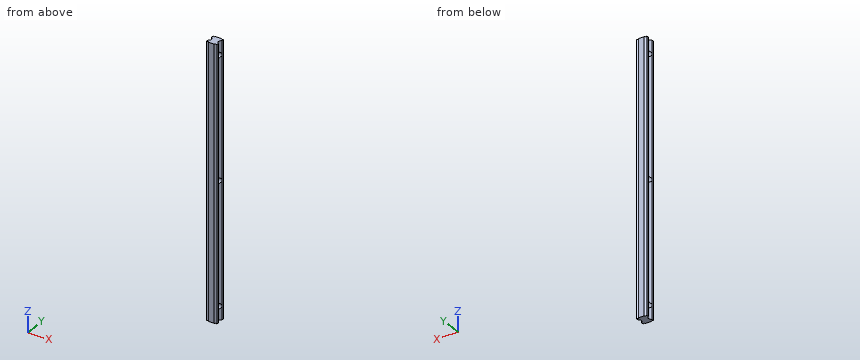
Autodesk Inventor part; units mm, degrees
ref_plane "to_ball_1_XY" through (1.2, -0.75, 109.375) normal (0, 0, 1) x (1, 0, 0)
ref_plane "to_ball_1_YZ" through (1.2, -0.75, 109.375) normal (1, 0, 0) x (0, 1, 0)
ref_plane "to_ball_1_ZX" through (1.2, -0.75, 109.375) normal (0, 1, 0) x (0, 0, 1)
sketch "Sketch_1" plane through (0, 0, 0) normal (0, 0, 1) x (1, 0, 0)
  line L0 (0, 2.9516) -> (0, 0.3457)
  arc A0 (2.6416, 0) -> (0, 0.3457) centre (1.2, -0.75) ccw
  line L1 (2.6416, 0) -> (8.7584, 0)
  arc A1 (11.4, 0.3457) -> (8.7584, 0) centre (10.2, -0.75) ccw
  line L2 (11.4, 0.3457) -> (11.4, 2.9516)
  arc A2 (11.4, 9.1484) -> (11.4, 2.9516) centre (12.8, 6.05) ccw
  line L3 (11.4, 9.1484) -> (11.4, 11.7543)
  arc A3 (8.7584, 12.1) -> (11.4, 11.7543) centre (10.2, 12.85) ccw
  line L4 (8.7584, 12.1) -> (2.6416, 12.1)
  arc A4 (0, 11.7543) -> (2.6416, 12.1) centre (1.2, 12.85) ccw
  line L5 (0, 11.7543) -> (0, 9.1484)
  arc A5 (0, 2.9516) -> (0, 9.1484) centre (-1.4, 6.05) ccw
extrude "Extrusion1" add sketch "Sketch_1" along normal blind 300
sketch "Sketch_3" plane through (0, 0, 15) normal (0, 0, 1) x (1, 0, 0)
  line L0 (11.4, 6.05) -> (0, 6.05)
  line L1 (0, 6.05) -> (0, 9.3)
  line L2 (0, 9.3) -> (11.4, 9.3)
  line L3 (11.4, 9.3) -> (11.4, 6.05)
  line L4 (11.4, 6.05) -> (0, 6.05)
revolve "Revolution1" cut sketch "Sketch_3" angle 360 about axis through (11.4, 6.05, 15) along (1, 0, 0)
pattern_linear "Rectangular Pattern1" count 3 spacing 135 along (0, 0, 1) of "Revolution1"
ref_plane "to_ball_1_XY" through (1.2, -0.75, 109.375) normal (0, 0, 1) x (1, 0, 0)
ref_plane "to_ball_1_YZ" through (1.2, -0.75, 109.375) normal (1, 0, 0) x (0, 1, 0)
ref_plane "to_ball_1_ZX" through (1.2, -0.75, 109.375) normal (0, 1, 0) x (0, 0, 1)
ref_plane "to_ball_2_XY" through (10.2, -0.75, 109.375) normal (0, 0, 1) x (1, 0, 0)
ref_plane "to_ball_2_YZ" through (10.2, -0.75, 109.375) normal (1, 0, 0) x (0, 1, 0)
ref_plane "to_ball_2_ZX" through (10.2, -0.75, 109.375) normal (0, 1, 0) x (0, 0, 1)
ref_plane "to_ball_3_XY" through (1.2, 12.85, 109.375) normal (0, 0, 1) x (1, 0, 0)
ref_plane "to_ball_3_YZ" through (1.2, 12.85, 109.375) normal (1, 0, 0) x (0, 1, 0)
ref_plane "to_ball_3_ZX" through (1.2, 12.85, 109.375) normal (0, 1, 0) x (0, 0, 1)
ref_plane "to_ball_4_XY" through (10.2, 12.85, 109.375) normal (0, 0, 1) x (1, 0, 0)
ref_plane "to_ball_4_YZ" through (10.2, 12.85, 109.375) normal (1, 0, 0) x (0, 1, 0)
ref_plane "to_ball_4_ZX" through (10.2, 12.85, 109.375) normal (0, 1, 0) x (0, 0, 1)
ref_plane "to_body_XY" through (5.6, 6.05, 150) normal (0, 0, 1) x (1, 0, 0)
ref_plane "to_body_YZ" through (5.6, 6.05, 150) normal (1, 0, 0) x (0, 1, 0)
ref_plane "to_body_ZX" through (5.6, 6.05, 150) normal (0, 1, 0) x (0, 0, 1)
ref_plane "to_body2_XY" through (5.8, 6.05, 150) normal (0, 0, 1) x (1, 0, 0)
ref_plane "to_body2_YZ" through (5.8, 6.05, 150) normal (1, 0, 0) x (0, 1, 0)
ref_plane "to_body2_ZX" through (5.8, 6.05, 150) normal (0, 1, 0) x (0, 0, 1)
properties part number "SAR330-30_r" material "Aluminum 6061"
Source: CAD feature listing. Evaluate the final solid. Frame: model axes, mm. Give positions to 0.01 mm unless a question says otherwise; leave off trailing zeros. Order: outer loops, then holes, each group sorted by start corner. A loop starts at its lowest first (then second) coordinate and runs counter-clockwise, first axis right, second up. Notation, with made-up numbers: (17.5, -11.75) -> (75.5, -11.75) arc R21 cw to (75.5, 11.25) -> close; hole circle Ø2 at (-5.5, -1). An arc over 180 degrees is marked (long way). Use a Markdown table: item, result.
Q1. First-contact query: P1, Ø5, axis at y = 6.05, z = 285, coming from the +X side. Flat tip, straight axial feed; report the tip coordinate or a pass-through.
A:
| item | result |
|---|---|
| P1 | through |
Q2. Section B-B (x = 6.5). Return the cut outline in (y, z).
A:
| item | result |
|---|---|
| outline | (0, 0) -> (12.1, 0) -> (12.1, 300) -> (0, 300) -> close; hole circle Ø6.5 at (6.05, 15); hole circle Ø6.5 at (6.05, 150); hole circle Ø6.5 at (6.05, 285) |
Q3. Material intervals for line 1 (Z direction, x = 7.25, y = 6.5); line 2 (Z direction, x = 9.25, y = 7.75); line 3 (Y direction, x = 6, z = 15), sorted ascending. Write a range as [from, to].
A:
| item | result |
|---|---|
| line 1 | [0, 11.78], [18.22, 146.78], [153.22, 281.78], [288.22, 300] |
| line 2 | [0, 12.23], [17.77, 147.23], [152.77, 282.23], [287.77, 300] |
| line 3 | [0, 2.8], [9.3, 12.1] |
Q4. Section A-A (y = 6.05). Return the cut outline in (x, z).
A:
| item | result |
|---|---|
| outline | (2, 0) -> (9.4, 0) -> (9.4, 11.75) -> (2, 11.75) -> close; (2, 18.25) -> (9.4, 18.25) -> (9.4, 146.75) -> (2, 146.75) -> close; (2, 153.25) -> (9.4, 153.25) -> (9.4, 281.75) -> (2, 281.75) -> close; (2, 288.25) -> (9.4, 288.25) -> (9.4, 300) -> (2, 300) -> close |
Q5. Section C-C (z = 29.5). Return the cut outline in (x, y), and give its area (3 significant figures).
A:
| item | result |
|---|---|
| outline | (0, 0.35) arc R1.62 cw to (2.64, 0) -> (8.76, 0) arc R1.63 cw to (11.4, 0.35) -> (11.4, 2.95) arc R3.4 cw to (11.4, 9.15) -> (11.4, 11.75) arc R1.62 cw to (8.76, 12.1) -> (2.64, 12.1) arc R1.63 cw to (0, 11.75) -> (0, 9.15) arc R3.4 cw to (0, 2.95) -> close |
| area | 113 mm^2 |
